Work out the finished part from the listing and answer in its coordinate system (mm). Face numbers are marked on the shaded views. A direction names the side the tool comes from. Coordinates: 2 decimals unless noted, no trailing zeros. Write each loop counter-clockwise with the first axis right and the second up, starting at its lowest first coordinate (ties: lowest second). Pieces come first, ordered by that corner, then holes. Notation, with made-up numbers: (43, -14.5) - (59, -14.5) arc R17 ccw to (59, -8.5) - close; hole circle Ø11 at (19.5, 52). An arc over 180 degrees is marked (long way). Use CSV: the item, a comma, the result in double quotes. Start each with the question number.
from build123d import *

# Parameters (mm, degrees)
BOSS_EXTRUDE1_DEPTH = 37.592
CUT_EXTRUDE1_DEPTH  = 37.592
SKETCH3_R           = 1.651
CUT_EXTRUDE3_DEPTH  = 37.592
CUT_EXTRUDE4_DEPTH  = 37.592
CUT_EXTRUDE5_DEPTH  = 37.592
SKETCH7_R           = 1.651
CUT_EXTRUDE6_DEPTH  = 37.592
LPATTERN1_COUNT     = 7
LPATTERN1_PITCH     = 6.35
CUT_EXTRUDE7_DEPTH  = 37.592


with BuildPart() as part:
    # Sketch1 → Boss-Extrude1 (new body)
    with BuildSketch(Plane.XY):
        Polygon((-1.016, 18.796), (1.016, 18.796), (1.016, -18.796), (50.292, -18.796), (50.292, -20.828), (-1.016, -20.828), (-1.016, -18.796), align=None)
    extrude(amount=-BOSS_EXTRUDE1_DEPTH)

    # Sketch2 → Cut-Extrude1 (cut)
    with BuildSketch(Plane.ZY.offset(1.016)):
        with BuildLine():
            Line((-25.4, -6.985), (-25.4, 6.985))
            ThreePointArc((-25.4, 6.985), (-18.796, 13.589), (-12.192, 6.985))
            Line((-12.192, 6.985), (-12.192, -6.985))
            ThreePointArc((-12.192, -6.985), (-18.796, -13.589), (-25.4, -6.985))
        make_face()
    extrude(amount=-CUT_EXTRUDE1_DEPTH, mode=Mode.SUBTRACT)

    # Sketch3 → Cut-Extrude3 (cut)
    with BuildSketch(Plane.ZY.offset(1.016)):
        with Locations((-34.29, 0)):
            Circle(SKETCH3_R)
        with Locations((-26.67, -13.344068345)):
            Circle(SKETCH3_R)
        with Locations((-10.922, -13.344068345)):
            Circle(SKETCH3_R)
        with Locations((-3.302, 0)):
            Circle(SKETCH3_R)
        with Locations((-10.922, 13.344068345)):
            Circle(SKETCH3_R)
        with Locations((-26.67, 13.344068345)):
            Circle(SKETCH3_R)
    extrude(amount=-CUT_EXTRUDE3_DEPTH, mode=Mode.SUBTRACT)

    # Sketch5 → Cut-Extrude4 (cut)
    with BuildSketch(Plane.ZY.offset(1.016)):
        with BuildLine():
            Line((-37.592, 18.796), (-37.592, -1.016))
            ThreePointArc((-37.592, -1.016), (-32.145348176, 12.638714937), (-18.796, 18.796))
            Line((-18.796, 18.796), (-37.592, 18.796))
        make_face()
        with BuildLine():
            Line((0, 18.796), (-16.915162607, 18.796))
            ThreePointArc((-16.915162607, 18.796), (-5.212279302, 13.583720698), (0, 1.880837393))
            Line((0, 1.880837393), (0, 18.796))
        make_face()
    extrude(amount=-CUT_EXTRUDE4_DEPTH, mode=Mode.SUBTRACT)

    # Sketch6 → Cut-Extrude5 (cut)
    with BuildSketch(Plane(origin=(0, -18.796, 0), x_dir=(1, 0, 0), z_dir=(0, 1, 0))):
        with BuildLine():
            Line((50.292, 2.413), (50.292, 0))
            Line((50.292, 0), (47.879, 0))
            ThreePointArc((47.879, 0), (49.585248663, 0.706751337), (50.292, 2.413))
        make_face()
    extrude(amount=-CUT_EXTRUDE5_DEPTH, mode=Mode.SUBTRACT)

    # Sketch7 → Cut-Extrude6 (cut)
    with BuildSketch(Plane(origin=(0, -18.796, 0), x_dir=(1, 0, 0), z_dir=(0, 1, 0))):
        with Locations((45.466, 3.175)):
            Circle(SKETCH7_R)
        with Locations((45.466, 34.417)):
            Circle(SKETCH7_R)
    cut_extrude6 = extrude(amount=-CUT_EXTRUDE6_DEPTH, mode=Mode.SUBTRACT)

    # LPattern1: Cut-Extrude6 ×7
    with Locations(*[(-i * LPATTERN1_PITCH, 0, 0) for i in range(1, LPATTERN1_COUNT)]):
        add(cut_extrude6, mode=Mode.SUBTRACT)

    # Sketch8 → Cut-Extrude7 (cut)
    with BuildSketch(Plane(origin=(0, -18.796, 0), x_dir=(1, 0, 0), z_dir=(0, 1, 0))):
        with BuildLine():
            Line((50.292, 35.052), (50.292, 37.592))
            Line((50.292, 37.592), (47.752, 37.592))
            ThreePointArc((47.752, 37.592), (49.548051224, 36.848051224), (50.292, 35.052))
        make_face()
    extrude(amount=-CUT_EXTRUDE7_DEPTH, mode=Mode.SUBTRACT)


solid = part.part
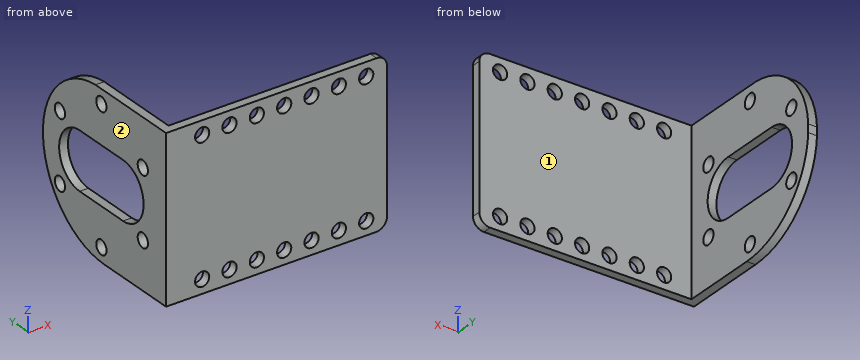
Item 1: Each of these flat-tipped pins is pushed along its axis until it touches: pin 1 (3 mm diameter, centred on x = 42, z = -14, fed in from +Y); pin 2 (5.5 mm diameter, centred on y = 0, z = -3.302, fed in from +X). Where does it stop, or does it pass through?
Item 2: A cutting plane is placed at C-C (z = -15). Determine the outline of the cut face in (x, y).
Item 3: Which of the six approach directions +Z, -Z, +X, -X, +Y, -Y give full straight-line access (tool end or side, diameter ignored) to the marked faces 1 and 2?
Item 4: A cutting plane is placed at B-B (x = 46). Determine the outline of the cut face in (y, z), then the cut area to 3 significant figures.
Item 5: Straight lines are drawn through the part: probe 1 along X at (y, z) = (12.5, -30.5); probe 2 along Y at (x, z) = (31, -27.5). For each, find the intervals that lie inside material, in ascending order. Write a range as [from, to].
Item 6: A cutting plane is placed at D-D (z = -26.67). Determine the outline of the cut face in (x, y), then the cut area to 3 significant figures.
Item 7: A cutting plane is placed at A-A (y = -4). Determine the outline of the cut face in (x, z).
Calculated:
1,pin 1,"stops at y = -18.8"
1,pin 2,"stops at x = 1.02"
2,outline,"(-1.02, -20.83) - (50.29, -20.83) - (50.29, -18.8) - (1.02, -18.8) - (1.02, -12.39) - (-1.02, -12.39) - close; (-1.02, 12.39) - (1.02, 12.39) - (1.02, 18.59) - (-1.02, 18.59) - close"
3,face 1,"+Z, -Z, +X, +Y"
3,face 2,"+Z, -Z, -X, +Y, -Y"
4,outline,"(-20.83, -37.59) - (-18.8, -37.59) - (-18.8, -35.98) - (-20.83, -35.98) - close; (-20.83, -32.85) - (-18.8, -32.85) - (-18.8, -4.74) - (-20.83, -4.74) - close; (-20.83, -1.61) - (-18.8, -1.61) - (-18.8, 0) - (-20.83, 0) - close"
4,area,"63.7 mm²"
5,probe 1,"x = [-1.02, 1.02]"
5,probe 2,"y = [-20.83, -18.8]"
6,outline,"(-1.02, -20.83) - (50.29, -20.83) - (50.29, -18.8) - (1.02, -18.8) - (1.02, -15) - (-1.02, -15) - close; (-1.02, -11.69) - (1.02, -11.69) - (1.02, 11.69) - (-1.02, 11.69) - close; (-1.02, 15) - (1.02, 15) - (1.02, 16.71) - (-1.02, 16.71) - close"
6,area,"163 mm²"
7,outline,"(-1.02, -37.59) - (1.02, -37.59) - (1.02, -25.4) - (-1.02, -25.4) - close; (-1.02, -12.19) - (1.02, -12.19) - (1.02, 0) - (-1.02, 0) - close"
